```python
from build123d import *

# Parameters (mm, degrees)
CHAMFER3_SIZE = 1


with BuildPart() as part:
    # Sketch1 → Revolve1 (revolve)
    with BuildSketch(Plane.XY):
        with BuildLine():
            Line((41.074068666, 14.752070976), (44.895002352, 25.25))
            Line((44.895002352, 25.25), (47.701702352, 25.25))
            Line((47.701702352, 25.25), (47.701702352, 23.1186))
            Line((47.701702352, 23.1186), (46.126902352, 22.450137059))
            Line((46.126902352, 22.450137059), (46.126902352, 21.187062941))
            Line((46.126902352, 21.187062941), (47.701702352, 20.5186))
            Line((47.701702352, 20.5186), (47.701702352, 9))
            Line((47.701702352, 9), (0, 9))
            Line((0, 9), (0, 14))
            Line((0, 14), (40, 14))
            ThreePointArc((40, 14), (40.655597867, 14.206709213), (41.074068666, 14.752070976))
        make_face()
    revolve(axis=Axis((0, 0, 0), (1, 0, 0)))

    # Chamfer3
    chamfer3_edges = [part.edges().sort_by_distance(p)[0] for p in [
        (0, -14, 0),
    ]]
    chamfer(chamfer3_edges, length=CHAMFER3_SIZE)


solid = part.part
```
The model under review builds one solid part; all positions refer to its coordinate system, in mm. Round coordinates to 2 decimals unless told otherwise and drop trailing zeros. Loops run counter-clockwise (first coordinate to the right, second up) from the corner with the lowest first, then second, coordinate; pieces in that order, holes last. Notation, with made-up numbers: (-17.5, 42) -> (1.5, 42) arc R22 cw to (1.5, 51) -> close; hole circle Ø3 at (4, 84.5). An arc over 180 degrees is marked (long way). Answer as a JSON object with one key per item and string values. Group by question number.
1) We need section A-A on z = 0. Write out the cut boundary in (x, y) (3 decimals).
2) We need section C-C on x = 4. Write out the cut boundary in (y, z), then the cut area to 3 significant figures.
3) Mouldability with a two-part tool opening along Y and no side actions: class faces 1 (the face through (46.127, 17, 13)), 2 (the face through (47.702, 9, -4)), 3 (the face through (20.773, 12.932, -5.362)) as released by +Y, released by -Y, zero draft, split by the parting line, or undercut.
4) For line 1 (Z direction, x = 33, y = 0); line 2 (Z direction, x = 7, y = 8); line 3 (X direction, y = 22, z = 2), list the stretches that pass through material, from the lowest coordinate up. Write a range as [from, to].
5) For pin 1 Ø1.5 at (x, y) = (35.5, 13.5) entering from +Z; pin 2 Ø8 at (x, y) = (26.5, 16) entering from +Z; pin 3 Ø8 at (x, y) = (33, 6) entering from +Z, all flat-tipped, find the tip position at first contact; note any pin that passes through.
Result set:
{
 "1": {"outline": "(0, -13) -> (1, -14) -> (40, -14) arc R1.143 cw to (41.074, -14.752) -> (44.895, -25.25) -> (47.702, -25.25) -> (47.702, -23.119) -> (46.127, -22.45) -> (46.127, -21.187) -> (47.702, -20.519) -> (47.702, -9) -> (0, -9) -> close; (0, 9) -> (47.702, 9) -> (47.702, 20.519) -> (46.127, 21.187) -> (46.127, 22.45) -> (47.702, 23.119) -> (47.702, 25.25) -> (44.895, 25.25) -> (41.074, 14.752) arc R1.143 cw to (40, 14) -> (1, 14) -> (0, 13) -> close"},
 "2": {"outline": "circle Ø28 at (0, 0); hole circle Ø18 at (0, 0)", "area": "361 mm²"},
 "3": {"face 1": "undercut", "face 2": "zero draft", "face 3": "split by the parting line"},
 "4": {"line 1": "[-14, -9], [9, 14]", "line 2": "[-11.49, -4.12], [4.12, 11.49]", "line 3": "[43.75, 46.13]"},
 "5": {"pin 1": "z = 5.78", "pin 2": "z = 7.21", "pin 3": "z = 13.86"}
}
